For this review, take the finished solid that the model builds, in its own axes (mm). A direction names the side the tool comes from. Coordinates: 2 decimals unless noted, no trailing zeros. Write each loop counter-clockwise with the first axis right and the second up, starting at its lowest first coordinate (ties: lowest second). Pieces come first, ordered by that corner, then holes. Notation, with made-up numbers: (-31, 23) - (-26, 23) arc R12 cw to (-26, 46) - close; hole circle Ø10 at (-35.5, -6). An arc over 180 degrees is marked (long way). Write each question's results on one line, items separated by ' | '.
Autodesk Inventor part; units mm, degrees
ref_plane "Work Plane1" through (0, 0, 0) normal (0, -1, 0) x (1, 0, 0)
ref_plane "YZ Plane" through (0, 0, 0) normal (1, 0, 0) x (0, 1, 0)
ref_plane "XZ Plane" through (0, 0, 0) normal (0, 1, 0) x (-1, 0, 0)
sketch "Sketch1" plane through (0, 0, 0) normal (0, 1, 0) x (-1, 0, 0)
  line L0 (0, 0) -> (-59.8, 0)
  arc A0 (-59.8, 0) -> (-69.8, -10) centre (-59.8, -10) ccw
  line L1 (0, -1.9) -> (-59.8, -1.9)
  arc A1 (-59.8, -1.9) -> (-67.9, -10) centre (-59.8, -10) ccw
  line L2 (0, 0) -> (0, -1.9)
  line L3 (-67.9, -10) -> (-69.8, -10)
  dimension "d4" = 10
  dimension "d5" = 69.8
  dimension "d6" = 1.9
extrude "Extrusion1" add sketch "Sketch1" along normal mid plane 22.6
sketch "Sketch3" plane through (0, 0, 0) normal (1, 0, 0) x (0, 1, 0)
  line L0 (-11.3, -0.5) -> (-8.1, -0.5)
  line L1 (-8.1, -0.5) -> (-8.1, -1.4)
  line L2 (-8.1, -1.4) -> (-11.3, -1.4)
  line L3 (-11.3, -1.4) -> (-11.3, -0.5)
  line L4 (-11.3, 0) -> (-11.3, -1.9) construction
  line L5 (-11.8, -1.9) -> (-7.6, -1.9)
  line L6 (-7.6, -1.9) -> (-7.6, 0)
  line L7 (-7.6, 0) -> (-11.8, 0)
  line L8 (-11.8, 0) -> (-11.8, -1.9)
  point P0 (0, 0)
  point P1 (-11.3, -0.95)
  dimension "d11" = 3.2
  dimension "d12" = 0.9
  dimension "d18" = 0.5
  dimension "d19" = 0.5
  dimension "d20" = 0.5
  dimension "d21" = 0.5
extrude "Extrusion2" cut sketch "Sketch3" along normal blind 60.1 contours L0 L1 L2 L3
sketch "Sketch3 outline for Extrusion3" plane through (0, 0, 0) normal (1, 0, 0) x (0, 1, 0)
  line L0 (-11.8, -1.9) -> (-7.6, -1.9)
  line L1 (-11.8, 0) -> (-11.8, -1.9)
  line L2 (-7.6, 0) -> (-11.8, 0)
  line L3 (-7.6, -1.9) -> (-7.6, 0)
extrude "Extrusion3" cut sketch "Sketch3 outline for Extrusion3" along normal blind 0.5 draft -45
mirror "Mirror1" about plane through (0, 0, 0) normal (0, 1, 0) of "Extrusion2", "Extrusion3"
ref_plane "Work Plane1" through (0, 0, 0) normal (0, -1, 0) x (1, 0, 0)
sketch "Sketch4" plane through (0, 0, 0) normal (0, -1, 0) x (1, 0, 0)
  line L0 (67.9, -10) -> (69.8, -10)
  arc A0 (69.571144, -10) -> (68.263474, -10) centre (68.917309, -10.25) ccw
  point P0 (0, 0)
  dimension "d26" = 0.7
  dimension "d27" = 0.25
extrude "Extrusion4" cut sketch "Sketch4" along normal mid plane 10.4
sketch "Sketch5" plane through (0, 0, 0) normal (0, 1, 0) x (-1, 0, 0)
  arc A0 (-4, 0) -> (-6, 0) centre (-5, 0) ccw
  line L0 (-6, 0) -> (-4, 0)
  line L1 (-59.8, 0) -> (0, 0) construction
  dimension "d30" = 1
  dimension "d31" = 5
extrude "Extrusion5" add sketch "Sketch5" along normal mid plane 10
equation "\"d4\" = fillet_outer_radius"
equation "\"d5\" = -fillet_outer_radius + total_width - 2 * tol"
equation "\"d6\" = thickness - tol"
equation "\"d7\" = door_height - 4 * tol"
equation "\"d11\" = door_rail_height + 2 * tol"
equation "\"d12\" = door_rail_depth + 4 * tol"
equation "\"d18\" = door_rail_depth"
equation "\"d19\" = door_rail_depth"
equation "\"d20\" = door_rail_depth"
equation "\"d21\" = door_rail_depth"
equation "\"d13\" = -2 * fillet_outer_radius + total_width + tol"
equation "\"d22\" = door_rail_depth"
equation "\"d26\" = door_strike_radius + 2 * tol"
equation "\"d28\" = door_strike_height + 4 * tol"
equation "\"d30\" = door_handle_radius"
equation "\"d31\" = door_handle_inset_width"
equation "\"d32\" = door_handle_height"
equation "\"door_handle_inset_width\" = 5"
equation "\"door_handle_height\" = 10"
equation "\"door_handle_radius\" = 1"
properties part number "DOOR" material "PC/ABS Plastic"
Q1. For faces 1 (the face through (30, -10, -1.4)), 2 (the face through (68.91, 0.07, -9.55)), 3 (the face through (5, 0, 1)), 4 (the face through (29, 0, -1.9)), 5 (the face through (30, 10, -0.5)), list the 3-axis set-ups (+Z, -Z, +X, -X, +Y, -Y) from which the entire face can be reached by the end or side of a thin tool; tool diameter is ignored.
Results found:
face 1: -X, -Y | face 2: -Z | face 3: +Z, +Y, -Y | face 4: -Z, -X, +Y, -Y | face 5: -X, +Y
Q2. Wall thickness on line 1 along Z through (x, y) = (36, -9.75); line 2 along Z through (x, y) = (17, 7.5); line 3 along Y through (x, z) = (58.5, -1.25): over which ranges is each line inside the solid? List them lowest first. Write a range as from..to.
Results found:
line 1: -1.9..-1.4, -0.5..0 | line 2: -1.9..0 | line 3: -8.1..8.1
Q3. Take a section at C-C on z = -8.75. State the section outline as (x, y) points, plus the area to 3 significant figures.
Results found:
outline: (67.8, -11.3) - (69.72, -11.3) - (69.72, 11.3) - (67.8, 11.3) - close | area: 43.4 mm2
Q4. Take a section at D-D on x = 5. State the section outline as (y, z) points, plus the area to 3 significant figures.
Results found:
outline: (-11.3, -1.9) - (11.3, -1.9) - (11.3, -1.4) - (8.1, -1.4) - (8.1, -0.5) - (11.3, -0.5) - (11.3, 0) - (5, 0) - (5, 1) - (-5, 1) - (-5, 0) - (-11.3, 0) - (-11.3, -0.5) - (-8.1, -0.5) - (-8.1, -1.4) - (-11.3, -1.4) - close | area: 47.2 mm2
Q5. Take a section at A-A on x = 23. State the section outline as (y, z) points, plus the area to 3 significant figures.
Results found:
outline: (-11.3, -1.9) - (11.3, -1.9) - (11.3, -1.4) - (8.1, -1.4) - (8.1, -0.5) - (11.3, -0.5) - (11.3, 0) - (-11.3, 0) - (-11.3, -0.5) - (-8.1, -0.5) - (-8.1, -1.4) - (-11.3, -1.4) - close | area: 37.2 mm2
Q6. Mouldability with a two-part tool opening along Z and no side actions: class faces 6 (the face through (29, 0, 0)), 7 (the face through (30, -10, -0.5)), 8 (the face through (42.8, -11.3, -1.6)) as pulls with the +Z half, pulls with the -Z half, needs draft (parallel to the pull), parting line crosses it, or undercut.
Results found:
face 6: pulls with the +Z half | face 7: undercut | face 8: needs draft
Q7. For pin 1 (1.5 mm diameter, centred on y = 4.5, z = -7.5, fed in from -X); pin 2 (3.5 mm diameter, centred on x = 17, y = 10, fed in from +Z); pin 3 (2.5 mm diameter, centred on x = 26.5, y = -10, fed in from -Z); pin 4 (5 mm diameter, centred on y = -1, z = -1, fed in from -X), all flat-tipped, find the tip position at first contact; note any pin that passes through.
Results found:
pin 1: x = 67.22 | pin 2: z = 0 | pin 3: z = -1.9 | pin 4: x = 0
Q8. Take a section at B-B on y = 3.75. State the section outline as (x, z) points, plus the area to 3 significant figures.
Results found:
outline: (0, -1.9) - (59.8, -1.9) arc R8.1 cw to (67.9, -10) - (68.26, -10) arc R0.7 cw to (69.57, -10) - (69.8, -10) arc R10 ccw to (59.8, 0) - (6, 0) arc R1 ccw to (4, 0) - (0, 0) - close | area: 142 mm2
